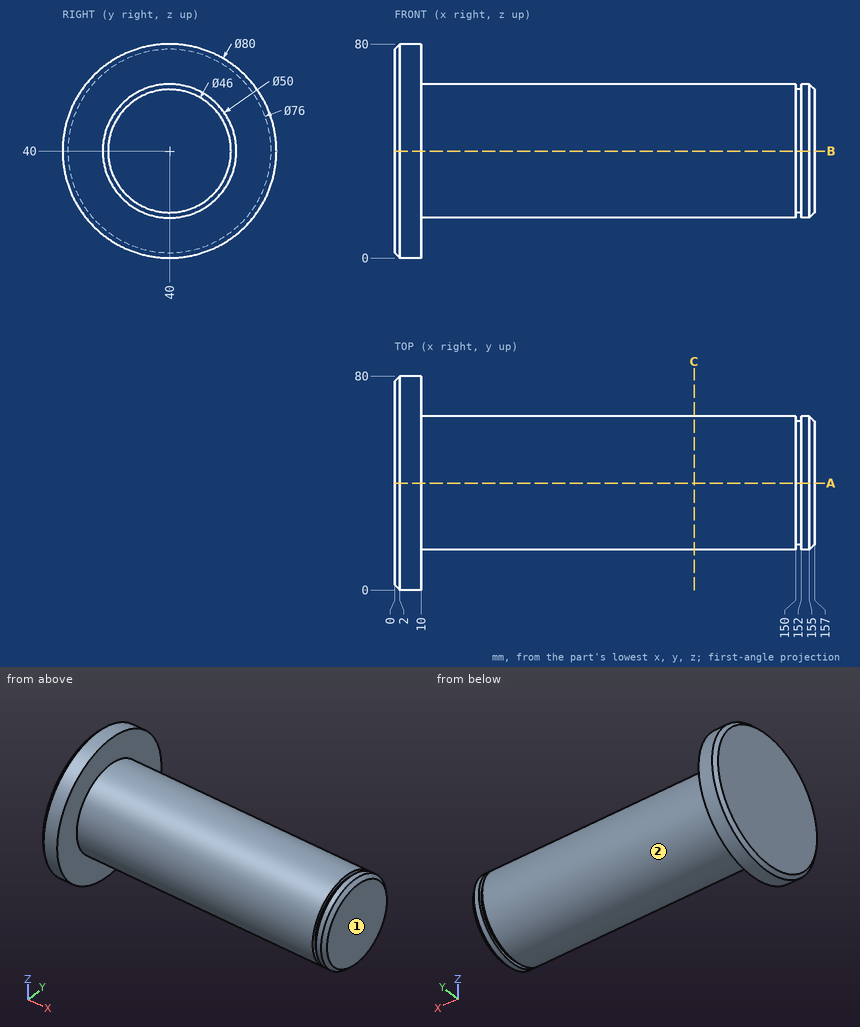
Print and shaded views of the part. All mm, measured from the part's lowest x, y and z. A direction names the side the tool comes from. Coordinates: 2 decimals unless noted, no trailing zeros. Write each loop counter-clockwise with the first axis right and the second up, starting at its lowest first coordinate (ties: lowest second). Pieces come first, ordered by that corner, then holes.
(1) Cut at C-C, the plane x = 112. List the corners of the cut face in (y, z).
(2) Drill centre lines: probe 1 along X at (y, z) = (15, 59.5); probe 2 along Y at (x, z) = (148, 39.5) (3 decimals); probe 3 along Y at (x, z) = (118.5, 18.5). Where is each one in solid material? Low to high.
(3) Flat gauge pins, fed straight in: pin 1 (2 mm diameter, centred on x = 116, y = 27.5, fed in from -Z); pin 2 (2 mm diameter, centred on x = 123.5, z = 16, fed in from +Y); pin 3 (3 mm diameter, centred on x = 93, y = 54.5, fed in from -Z). Where does each tip first touch, or does it go through?
(4) 3-axis set-ups, long thin cutter, end or side, ignore diameter. For the marked faces 1 and 2: which of +Z, -Z, +X, -X, +Y, -Y reach the whole face in a straight line?
(5) Cut at A-A, the plane y = 40. List the corners of the cut face in (x, z), and give its area (3 significant figures).
Geometry says:
1. outline: circle Ø50 at (40, 40)
2. probe 1: x = 0 to 10
2. probe 2: y = 15.005 to 64.995
2. probe 3: y = 27.24 to 52.76
3. pin 1: stops at z = 17.8
3. pin 2: stops at y = 49.8
3. pin 3: stops at z = 18.65
4. face 1: +Z, -Z, +X, +Y, -Y
4. face 2: +X
5. outline: (0, 2) - (2, 0) - (10, 0) - (10, 15) - (150, 15) - (150, 17) - (152, 17) - (152, 15) - (155, 15) - (157, 17) - (157, 63) - (155, 65) - (152, 65) - (152, 63) - (150, 63) - (150, 65) - (10, 65) - (10, 80) - (2, 80) - (0, 78) - close
5. area: 8,130 mm2
